```python
from build123d import *

# Parameters (mm, degrees)
SKETCH1_W                                        = 17.4625
SKETCH1_H                                        = 25.4
BOSS_EXTRUDE1_DEPTH                              = 12.7
SKETCH2_W                                        = 15.875
SKETCH2_H                                        = 1.5875
CUT_EXTRUDE1_DEPTH                               = 34.3375
F_8_32_TAPPED_HOLE1_D                            = 3.4544
F_8_32_TAPPED_HOLE1_DEPTH                        = 12.446
F_8_32_TAPPED_HOLE1_TIP                          = 1.037806461
CBORE_FOR_1_4_SOCKET_HEAD_CAP_SCREW1_D           = 7.14248
CBORE_FOR_1_4_SOCKET_HEAD_CAP_SCREW1_CBORE_D     = 11.1125
CBORE_FOR_1_4_SOCKET_HEAD_CAP_SCREW1_CBORE_DEPTH = 6.35


with BuildPart() as part:
    # Sketch1 → Boss-Extrude1 (new body)
    with BuildSketch(Plane.XY):
        with Locations((8.73125, 12.7)):
            Rectangle(SKETCH1_W, SKETCH1_H)
    extrude(amount=BOSS_EXTRUDE1_DEPTH)

    # Sketch2 → Cut-Extrude1 (cut, through all)
    with BuildSketch(Plane(origin=(0, 25.4, 0), x_dir=(1, 0, 0), z_dir=(0, 1, 0))):
        with Locations((9.525, -0.79375)):
            Rectangle(SKETCH2_W, SKETCH2_H)
    extrude(amount=-CUT_EXTRUDE1_DEPTH, mode=Mode.SUBTRACT)

    # #8-32 Tapped Hole1
    with Locations(Plane(origin=(17.4625, 0, 0), x_dir=(0, 0, -1), z_dir=(1, 0, 0))):
        with Locations((-7.9375, 16.66875), (-7.9375, 8.73125)):
            Hole(F_8_32_TAPPED_HOLE1_D / 2, depth=F_8_32_TAPPED_HOLE1_DEPTH)
            with Locations((0, 0, -(F_8_32_TAPPED_HOLE1_DEPTH + F_8_32_TAPPED_HOLE1_TIP / 2))):  # 118° drill point
                Cone(0, F_8_32_TAPPED_HOLE1_D / 2, F_8_32_TAPPED_HOLE1_TIP, mode=Mode.SUBTRACT)

    # CBORE for 1/4 Socket Head Cap Screw1 (through all)
    with Locations(Plane.XY.offset(12.7)):
        with Locations((11.1125, 12.7)):
            CounterBoreHole(CBORE_FOR_1_4_SOCKET_HEAD_CAP_SCREW1_D / 2, CBORE_FOR_1_4_SOCKET_HEAD_CAP_SCREW1_CBORE_D / 2, CBORE_FOR_1_4_SOCKET_HEAD_CAP_SCREW1_CBORE_DEPTH)


solid = part.part
```
Work out the finished part from the listing and answer in its coordinate system (mm). A direction names the side the tool comes from. Round coordinates to 2 decimals unless told otherwise and drop trailing zeros. Write each loop counter-clockwise with the first axis right and the second up, starting at its lowest first coordinate (ties: lowest second). Pieces come first, ordered by that corner, then holes. Notation, with made-up numbers: (-14.5, -18.5) -> (29.5, -18.5) arc R22 cw to (29.5, 11.5) -> close; hole circle Ø7 at (23.5, -22). An arc over 180 degrees is marked (long way). Write each question's results on one line, items separated by ' | '.
1) Which of the six approach directions +Z, -Z, +X, -X, +Y, -Y give full straight-line access (tool end or side, diameter ignored) to faces 5 (the flat face through (5, 13, 12.7)), 6 (the flat face through (11.1, 7.7, 6.35)), 7 (the cylindrical face through (11.15, 18.38, 7.71)), 8 (the flat face through (1.588, 13, 1)), 9 (the flat face through (9, 0, 6))?
Findings:
face 5: +Z, +X, -X, +Y, -Y | face 6: +Z | face 7: +X | face 8: -Z, +X, +Y, -Y | face 9: +Z, -Z, +X, -X, -Y
2) For a pull along X with two mould halves and no side action, classify faces 1 (the cylindrical face through (11.158, 18.256, 6.713)), 2 (the flat face through (8, 10, 1.588)), 3 (the flat face through (17.462, 13, 7)), 4 (the flat face through (0, 13, 6)) as +X half, -X half, draft (parallel to the pull), parting line (faces both ways), or undercut.
Findings:
face 1: undercut | face 2: draft | face 3: +X half | face 4: -X half
3) The part is cut by section B-B (y = 12.7). Write down the section's boundary in (x, z), and give its area (3 significant figures).
Findings:
outline: (0, 0) -> (1.59, 0) -> (1.59, 1.59) -> (7.54, 1.59) -> (7.54, 6.35) -> (5.56, 6.35) -> (5.56, 12.7) -> (0, 12.7) -> close; (14.68, 1.59) -> (17.46, 1.59) -> (17.46, 12.7) -> (16.67, 12.7) -> (16.67, 6.35) -> (14.68, 6.35) -> close | area: 92.0 mm²
4) Flat-ended cylindrical pins translate along their axes: pin 1 (1.5 mm diameter, centred on x = 2.5, y = 15.5, fed in from -Z); pin 2 (0.8 mm diameter, centred on y = 15, z = 0.5, fed in from +X); pin 3 (9.5 mm diameter, centred on x = 11.11, y = 12.7, fed in from +Z). Find the tip coordinate at first contact, or state that the pin passes through.
Findings:
pin 1: stops at z = 1.59 | pin 2: stops at x = 1.59 | pin 3: stops at z = 6.35
5) The part is cut by section A-A (x = 10). Write down the section's boundary in (y, z), and give its area (3 significant figures).
Findings:
outline: (0, 1.59) -> (9.31, 1.59) -> (9.31, 6.31) arc R1.73 cw to (8.05, 6.35) -> (7.26, 6.35) -> (7.26, 7.04) arc R1.73 cw to (7.26, 8.84) -> (7.26, 12.7) -> (0, 12.7) -> close; (16.09, 1.59) -> (25.4, 1.59) -> (25.4, 12.7) -> (18.14, 12.7) -> (18.14, 8.84) arc R1.73 cw to (18.14, 7.04) -> (18.14, 6.35) -> (17.35, 6.35) arc R1.73 cw to (16.09, 6.31) -> close | area: 180 mm²
6) The part is cut by section C-C (z = 4.75). Write down the section's boundary in (x, y), and give its area (3 significant figures).
Findings:
outline: (0, 0) -> (17.46, 0) -> (17.46, 25.4) -> (0, 25.4) -> close; hole circle Ø7.14 at (11.11, 12.7) | area: 403 mm²
7) The part is cut by section D-D (z = 11.75). Write down the section's boundary in (x, y).
Findings:
outline: (0, 0) -> (17.46, 0) -> (17.46, 25.4) -> (0, 25.4) -> close; hole circle Ø11.11 at (11.11, 12.7)
8) Consider line 1 along X through (y, z) = (12.7, 2.9); line 2 along X through (y, z) = (12.5, 9.5); line 3 along X through (y, z) = (8.25, 1.5). Determine where each line is inside the solid, lowest interval first. Write a range as [from, to].
Findings:
line 1: x = [0, 7.54], [14.68, 17.46] | line 2: x = [0, 5.56], [16.67, 17.46] | line 3: x = [0, 1.59]
